The listing builds one solid part. Answer for the finished solid, in the listing's coordinates (mm). A direction names the side the tool comes from. Coordinates: 2 decimals unless noted, no trailing zeros. Write each loop counter-clockwise with the first axis right and the second up, starting at its lowest first coordinate (ties: lowest second). Pieces come first, ordered by that corner, then holes.
```python
from build123d import *

# Parameters (mm, degrees)
SKETCH2_R          = 1.35
CUT_EXTRUDE1_DEPTH = 10


with BuildPart() as part:
    # Sketch1 → Revolve1 (revolve)
    with BuildSketch(Plane.XY):
        Polygon((-5.298096504, 7), (-5.298096504, 12.715801809), (-2.708631043, 16.6), (9.701368957, 16.6), (9.701368957, 18.6), (11.701368957, 18.6), (11.701368957, 17.75), (10.701368957, 17.75), (10.701368957, 15.604601484), (4.215618846, 15.604601484), (2.715618846, 14.6), (-1.638263526, 14.6), (-2.798096504, 12.860250534), (-2.798096504, 7), align=None)
    revolve(axis=Axis((-25, 0, 0), (1, 0, 0)))

    # Sketch2 → Cut-Extrude1 (cut)
    with BuildSketch(Plane(origin=(-2.798096504, 0, 0), x_dir=(0, 0, -1), z_dir=(1, 0, 0))):
        with Locations((0, 9.5)):
            Circle(SKETCH2_R)
        with Locations((6.717514421, 6.717514421)):
            Circle(SKETCH2_R)
        with Locations((9.5, 0)):
            Circle(SKETCH2_R)
        with Locations((6.717514421, -6.717514421)):
            Circle(SKETCH2_R)
        with Locations((0, -9.5)):
            Circle(SKETCH2_R)
        with Locations((-6.717514421, -6.717514421)):
            Circle(SKETCH2_R)
        with Locations((-9.5, 0)):
            Circle(SKETCH2_R)
        with Locations((-6.717514421, 6.717514421)):
            Circle(SKETCH2_R)
    extrude(amount=-CUT_EXTRUDE1_DEPTH, mode=Mode.SUBTRACT)


solid = part.part
```
(1) Each of these flat-tipped pins is pushed along its axis until it touches: pin 1 (4.5 mm diameter, centred on y = 9.5, z = 0, fed in from +X); pin 2 (4 mm diameter, centred on y = 10.5, z = 14.5, fed in from -X); pin 3 (10 mm diameter, centred on y = -0.5, z = -10, fed in from +X). Where does it stop, or does it pass through?
(2) Section A-A, the plane y = 0 is taken. State how many separate pieces and enclosed holes the cut face has, plus the area to 3 significant figures.
(3) Find the intervals of material crossed by probe 1 along Z at (x, y) = (0.65, 0); probe 2 along Y at (x, z) = (4.5, 0.5); probe 3 along Z at (x, y) = (11.3, 0), in increasing order.
(4) Section C-C, the plane x = 7 is taken. Write down the section's boundary in (y, z).
(5) Which of the six approach directions +Z, -Z, +X, -X, +Y, -Y give full straight-line access (tool end or side, diameter ignored) to faces 1 (the cylindrical face through (-4.031, -8.161, 0.176)), 2 (the flat face through (-2.798, 5.5, -5.5)), 3 (the flat face through (9.701, 6.98, 15.24))?
(6) For a pull along Z with two mould halves and no side action, classify faces 4 (the flat face through (11.701, 10, -15)), 5 (the cylindrical face through (-4.031, -0.517, 8.253)), 6 (the cylindrical face through (3.583, -3.599, -16.205)) as pulls with the +Z half, pulls with the -Z half, needs draft (parallel to the pull), parting line crosses it, or undercut.
Solution:
1. pin 1: stops at x = -2.8
1. pin 2: stops at x = -3.17
1. pin 3: stops at x = 3.33
2. separate pieces: 4
2. enclosed holes: 0
2. area: 71.6 mm2
3. probe 1: z = -16.6 to -14.6, 14.6 to 16.6
3. probe 2: y = -16.59 to -15.6, 15.6 to 16.59
3. probe 3: z = -18.6 to -17.75, 17.75 to 18.6
4. outline: circle Ø33.2 at (0, 0); hole circle Ø31.21 at (0, 0)
5. face 1: +X, -X
5. face 2: +X
5. face 3: -X
6. face 4: needs draft
6. face 5: undercut
6. face 6: parting line crosses it
